For this review, use the dimensioned drawing (mm, ordinates from the lowest corner) and the shaded views. A direction names the side the tool comes from. Give positions to 0.01 mm unless a question says otherwise; leave off trailing zeros. Loops run counter-clockwise (first coordinate to the right, second up) from the corner with the lowest first, then second, coordinate; pieces in that order, holes last. Notation, with made-up numbers: M 8.5,12 L 52.5,12 A15 ccw 52.5,22 Z; hole C 77,-10 d3. An arc over 180 degrees is marked long. Use a Markdown table: item, result. Add a question column.
(1) Add section D-D, the plane x = 45. Give the boundary of the cut face in (y, z).
(2) Add section A-A, the plane y = 35. Give the boundary of the cut face in (x, z), then the cut area to 3 significant figures.
(3) Insertion check: pin 1 Ø6 at (y, z) = (55.5, 144) entering from -X; pin 2 Ø5 at (x, y) = (54.5, 17) entering from +Z; pin 3 Ø6 at (x, z) = (36.5, 168) entering from +Y. Each pin has a flat end and moves straight along its axis. Give the tip position at first contact, or say it passes through.
(4) Add section C-C, the plane z = 98. Give the boundary of the cut face in (x, y).
(5) Draft analysis for pull direction X (two halves, no side actions). For the marked faces 1 and 2, state which applies: pulls with the +X half, pulls with the -X half, needs draft (parallel to the pull), parting line crosses it, or undercut.
(6) For the marked faces 3, 4 and 5, list the 3-axis set-ups (+Z, -Z, +X, -X, +Y, -Y) from which the entire face can be reached by the end or side of a thin tool; tool diameter is ignored.
(7) For probe 1 along Z at (x, y) = (27, 62.5); probe 2 along Z at (x, y) = (30.5, 31.5); probe 3 along Y at (x, z) = (33, 85.5), list the stretches that pass through material, from the lowest coordinate up.
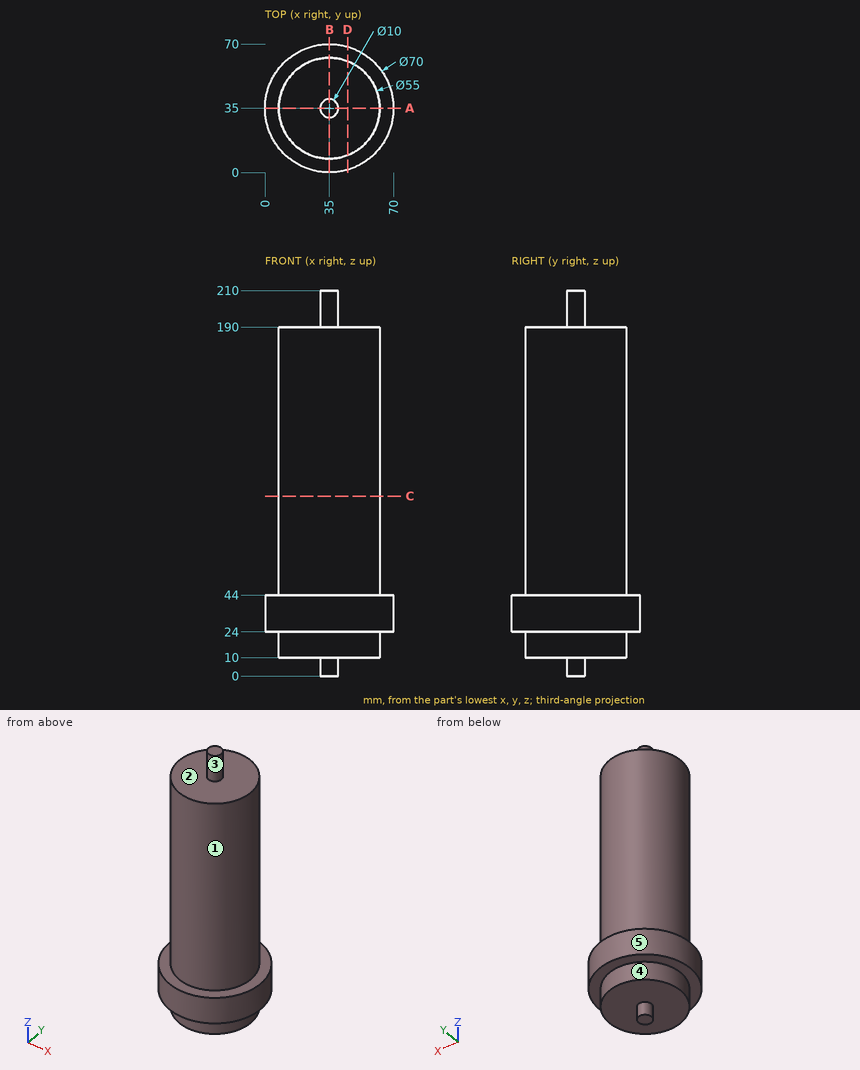
Established:
| question | item | result |
|---|---|---|
| 1 | outline | M 1.46,24 L 9.38,24 L 9.38,10 L 60.62,10 L 60.62,24 L 68.54,24 L 68.54,44 L 60.62,44 L 60.62,190 L 9.38,190 L 9.38,44 L 1.46,44 Z |
| 2 | outline | M 0,24 L 7.5,24 L 7.5,10 L 30,10 L 30,0 L 40,0 L 40,10 L 62.5,10 L 62.5,24 L 70,24 L 70,44 L 62.5,44 L 62.5,190 L 40,190 L 40,210 L 30,210 L 30,190 L 7.5,190 L 7.5,44 L 0,44 Z |
| 2 | area | 10,500 mm^2 |
| 3 | pin 1 | x = 13.79 |
| 3 | pin 2 | z = 190 |
| 3 | pin 3 | y = 62.5 |
| 4 | outline | C 35,35 d55 |
| 5 | face 1 | parting line crosses it |
| 5 | face 2 | needs draft |
| 6 | face 3 | +Z |
| 6 | face 4 | -Z |
| 6 | face 5 | +Z, -Z |
| 7 | probe 1 | 24 to 44 |
| 7 | probe 2 | 10 to 190 |
| 7 | probe 3 | 7.57 to 62.43 |
